Autodesk Inventor part; units mm, degrees
sketch "Sketch1" plane through (0, 0, 0) normal (0, 0, 1) x (1, 0, 0)
  line L0 (0, 1.6506) -> (0, -1.6506) construction
  line L1 (-3.3363, 0) -> (3.3363, 0) construction
  circle A0 centre (-22.86, -5.25) radius 2
  circle A1 centre (22.86, -5.25) radius 2
  circle A2 centre (0, 0) radius 2
  circle A3 centre (-35, -24) radius 2
  circle A4 centre (21, -24) radius 2
  circle A5 centre (35, -24) radius 2
  line L2 (-36.6788, -22.913) -> (-24.5388, -4.163)
  line L3 (-21.1812, -6.337) -> (-33.3212, -25.087)
  line L4 (33.3212, -25.087) -> (21.1812, -6.337)
  line L5 (24.5388, -4.163) -> (36.6788, -22.913)
  line L6 (23.3077, -3.3007) -> (0.4477, 1.9493)
  line L7 (-22.4123, -7.1993) -> (0.4477, -1.9493)
  line L8 (-23.3077, -3.3007) -> (-0.4477, 1.9493)
  line L9 (-0.4477, -1.9493) -> (22.4123, -7.1993)
  line L10 (19.0098, -23.8026) -> (20.8698, -5.0526)
  line L11 (22.9902, -24.1974) -> (24.8502, -5.4474)
  point P0 (19.0231, -24.3028)
  point P1 (1.0254, -1.7172)
  point P2 (-21.6219, -7.0177)
  point P3 (0, 3.0781)
  point P4 (22.9979, -23.9085)
  point P5 (21.6219, -7.0177)
  point P6 (24.2863, -11.1327)
  point P7 (20.6959, -6.8051)
  dimension "d0" = 45.72
  dimension "d1" = 22.86
  dimension "d4" = 4
  dimension "d5" = 4
  dimension "d6" = 4
  dimension "d7" = 18.75
  dimension "d8" = 18.75
  dimension "d9" = 14
  dimension "d10" = 18.75
  dimension "d11" = 56
  dimension "d12" = 70
  dimension "d13" = 35
  dimension "d14" = 4
  dimension "d15" = 4
  dimension "d16" = 4
  dimension "d34" = 5.25
  dimension "d35" = 5.25
extrude "Extrusion1" add sketch "Sketch1" along normal blind 2.4
sketch "Sketch2" plane through (0, 0, 2.4) normal (0, 0, 1) x (1, 0, 0)
  line L0 (-21.6219, -7.0177) -> (-33.3212, -25.087)
  arc A0 (-36.6788, -22.913) -> (-33.3212, -25.087) centre (-35, -24) ccw
  line L1 (-36.6788, -22.913) -> (-24.5388, -4.163)
  arc A1 (-23.3077, -3.3007) -> (-24.5388, -4.163) centre (-22.86, -5.25) ccw
  line L2 (-23.3077, -3.3007) -> (-0.4477, 1.9493)
  line L3 (24.5388, -4.163) -> (36.6788, -22.913)
  arc A2 (33.3212, -25.087) -> (36.6788, -22.913) centre (35, -24) ccw
  line L4 (33.3212, -25.087) -> (24.2863, -11.1327)
  line L5 (0, -2.0521) -> (-21.6219, -7.0177)
  arc A3 (19.0098, -23.8026) -> (22.9902, -24.1974) centre (21, -24) ccw
  line L6 (0.4477, 1.9493) -> (23.3077, -3.3007)
  arc A4 (24.5388, -4.163) -> (23.3077, -3.3007) centre (22.86, -5.25) ccw
  arc A5 (0.4477, 1.9493) -> (-0.4477, 1.9493) centre (0, 0) ccw
  line L7 (20.6959, -6.8051) -> (0, -2.0521)
  line L8 (24.2863, -11.1327) -> (22.9902, -24.1974)
  line L9 (19.0098, -23.8026) -> (20.6959, -6.8051)
hole "Hole1" at (-35, -24, 2.4) at (21, -24, 2.4) at (35, -24, 2.4) direction (0, 0, -1) diameter 2.8 depth 2.4
sketch "Sketch3" plane through (0, 0, 2.4) normal (0, 0, 1) x (1, 0, 0)
  circle A0 centre (35, -24) radius 1.4
  circle A1 centre (21, -24) radius 1.4
  circle A2 centre (-35, -24) radius 1.4
  line L0 (-21.6219, -7.0177) -> (-33.3212, -25.087)
  arc A3 (-36.6788, -22.913) -> (-33.3212, -25.087) centre (-35, -24) ccw
  line L1 (-36.6788, -22.913) -> (-24.5388, -4.163)
  arc A4 (-23.3077, -3.3007) -> (-24.5388, -4.163) centre (-22.86, -5.25) ccw
  line L2 (-23.3077, -3.3007) -> (-0.4477, 1.9493)
  line L3 (24.5388, -4.163) -> (36.6788, -22.913)
  arc A5 (33.3212, -25.087) -> (36.6788, -22.913) centre (35, -24) ccw
  line L4 (33.3212, -25.087) -> (24.2863, -11.1327)
  line L5 (0, -2.0521) -> (-21.6219, -7.0177)
  arc A6 (19.0098, -23.8026) -> (22.9902, -24.1974) centre (21, -24) ccw
  line L6 (0.4477, 1.9493) -> (23.3077, -3.3007)
  arc A7 (24.5388, -4.163) -> (23.3077, -3.3007) centre (22.86, -5.25) ccw
  arc A8 (0.4477, 1.9493) -> (-0.4477, 1.9493) centre (0, 0) ccw
  line L7 (20.6959, -6.8051) -> (0, -2.0521)
  line L8 (24.2863, -11.1327) -> (22.9902, -24.1974)
  line L9 (19.0098, -23.8026) -> (20.6959, -6.8051)
  circle A9 centre (-22.86, -5.25) radius 5
  circle A10 centre (0, 0) radius 4
  circle A11 centre (22.86, -5.25) radius 5
  dimension "d36" = 10
  dimension "d37" = 8
  dimension "d38" = 10
extrude "Extrusion3" add sketch "Sketch3" against normal up to surface (2.4 mm away) contours L5 A9 L0 | L0 A9 L1 A4 L2 L5 | A9 L2 A4 L1 | A10 L2 A8 L6 L7 L5 | L5 L7 A10 | A10 L6 A8 L2 | A11 L6 A7 L3 L9 L7 | L7 L9 A11 | A11 L3 A7 L6
sketch "Sketch4" plane through (0, 0, 0) normal (0, 0, -1) x (-1, 0, 0)
  arc A0 (-2.9285, -2.7246) -> (2.9285, -2.7246) centre (0, 0) ccw
  line L0 (-2.9285, -2.7246) -> (-17.946, -6.1735)
  arc A1 (-20.4174, -9.6128) -> (-17.946, -6.1735) centre (-22.86, -5.25) ccw
  line L1 (-20.4174, -9.6128) -> (-19.0098, -23.8026)
  arc A2 (-22.9902, -24.1974) -> (-19.0098, -23.8026) centre (-21, -24) ccw
  line L2 (-22.9902, -24.1974) -> (-24.2863, -11.1327)
  line L3 (-24.2863, -11.1327) -> (-33.3212, -25.087)
  arc A3 (-36.6788, -22.913) -> (-33.3212, -25.087) centre (-35, -24) ccw
  line L4 (-36.6788, -22.913) -> (-27.0294, -8.0097)
  arc A4 (-18.8414, -2.275) -> (-27.0294, -8.0097) centre (-22.86, -5.25) ccw
  line L5 (-18.8414, -2.275) -> (-3.8239, 1.1739)
  arc A5 (3.8239, 1.1739) -> (-3.8239, 1.1739) centre (0, 0) ccw
  line L6 (3.8239, 1.1739) -> (18.8414, -2.275)
  arc A6 (27.0294, -8.0097) -> (18.8414, -2.275) centre (22.86, -5.25) ccw
  line L7 (27.0294, -8.0097) -> (36.6788, -22.913)
  arc A7 (33.3212, -25.087) -> (36.6788, -22.913) centre (35, -24) ccw
  line L8 (33.3212, -25.087) -> (23.6718, -10.1837)
  arc A8 (17.946, -6.1735) -> (23.6718, -10.1837) centre (22.86, -5.25) ccw
  line L9 (17.946, -6.1735) -> (2.9285, -2.7246)
  circle A9 centre (-21, -24) radius 1.4
  circle A10 centre (-35, -24) radius 1.4
  circle A11 centre (35, -24) radius 1.4
hole "Hole3" at (-22.86, -5.25, 0) at (22.86, -5.25, 0) direction (0, 0, 1) diameter 3.3 depth 2.4 countersink diameter 6 countersink angle 90
sketch "Sketch5" plane through (0, 0, 2.4) normal (0, 0, 1) x (1, 0, 0)
  circle A0 centre (22.86, -5.25) radius 1.65
  circle A1 centre (-22.86, -5.25) radius 1.65
  arc A2 (-2.9285, -2.7246) -> (2.9285, -2.7246) centre (0, 0) ccw
  line L0 (-2.9285, -2.7246) -> (-17.946, -6.1735)
  arc A3 (-23.6718, -10.1837) -> (-17.946, -6.1735) centre (-22.86, -5.25) ccw
  line L1 (-23.6718, -10.1837) -> (-33.3212, -25.087)
  arc A4 (-36.6788, -22.913) -> (-33.3212, -25.087) centre (-35, -24) ccw
  line L2 (-36.6788, -22.913) -> (-27.0294, -8.0097)
  arc A5 (-18.8414, -2.275) -> (-27.0294, -8.0097) centre (-22.86, -5.25) ccw
  line L3 (-18.8414, -2.275) -> (-3.8239, 1.1739)
  arc A6 (3.8239, 1.1739) -> (-3.8239, 1.1739) centre (0, 0) ccw
  line L4 (3.8239, 1.1739) -> (18.8414, -2.275)
  arc A7 (27.0294, -8.0097) -> (18.8414, -2.275) centre (22.86, -5.25) ccw
  line L5 (27.0294, -8.0097) -> (36.6788, -22.913)
  arc A8 (33.3212, -25.087) -> (36.6788, -22.913) centre (35, -24) ccw
  line L6 (33.3212, -25.087) -> (24.2863, -11.1327)
  line L7 (24.2863, -11.1327) -> (22.9902, -24.1974)
  arc A9 (19.0098, -23.8026) -> (22.9902, -24.1974) centre (21, -24) ccw
  line L8 (19.0098, -23.8026) -> (20.4174, -9.6128)
  arc A10 (17.946, -6.1735) -> (20.4174, -9.6128) centre (22.86, -5.25) ccw
  line L9 (17.946, -6.1735) -> (2.9285, -2.7246)
  circle A11 centre (21, -24) radius 1.4
  circle A12 centre (35, -24) radius 1.4
  circle A13 centre (-35, -24) radius 1.4
hole "Hole4" at (0, 0, 2.4) direction (0, 0, -1) diameter 3.3 depth 2.4
properties part number "PD_Sensor" material "S235"
Design review of the part built by this model. Coordinates are the model's own, in mm. A direction names the side the tool comes from. Give positions to 0.01 mm unless a question says otherwise; leave off trailing zeros. Write each loop counter-clockwise with the first axis right and the second up, starting at its lowest first coordinate (ties: lowest second). Pieces come first, ordered by that corner, then holes.
(1) Mouldability with a two-part tool opening along X and no side actions: class faces 4 (the face through (31.79, -15.36, 1.18)), 5 (the face through (-31.922, -15.566, 1.183)), 6 (the face through (10.332, -4.425, 1.183)), 7 (the face through (-10.542, -4.473, 1.183)) as +X half, -X half, draft (parallel to the pull), parting line (faces both ways), or undercut.
Checked values:
face 4: +X half
face 5: -X half
face 6: undercut
face 7: undercut
(2) Add section B-B (x = -22.86). Give the boundary of the cut face in (y, z).
Checked values:
outline: (-10.25, 0) - (-8.25, 0) - (-6.9, 1.35) - (-6.9, 2.4) - (-10.25, 2.4) - close; (-3.6, 1.35) - (-2.25, 0) - (-0.25, 0) - (-0.25, 2.4) - (-3.6, 2.4) - close
(3) Tool access review of faces 1 (the face through (18.78, -8.14, 1.22)), 2 (the face through (-28.43, -17.53, 1.18)), 3 (the face through (11.438, -0.575, 1.183)): name each direction out of +Z, -Z, +X, -X, +Y, -Y from which nothing blocks a thin tool from reaching the whole face with its end or side.
Checked values:
face 1: +Z, -Z
face 2: +Z, -Z, -Y
face 3: +Z, -Z, +Y
(4) Wall thickness on line 1 along X through (y, z) = (-24, 1.9); line 2 along Y through (x, z) = (-22.86, 2.1); line 3 along X through (y, z) = (-22, 0.7): over which ranges is each line inside the solid? List them lowest first.
Checked values:
line 1: x = -37 to -36.4, -33.6 to -32.62, 19 to 19.6, 22.4 to 23.01, 32.62 to 33.6, 36.4 to 37
line 2: y = -10.25 to -6.9, -3.6 to -0.25
line 3: x = -36.09 to -31.32, 19.19 to 23.21, 31.32 to 36.09
(5) Add section D-D (y = -5.25). Give the boundary of the cut face in (x, z), and give its area (3 significant figures).
Checked values:
outline: (-27.86, 0) - (-25.86, 0) - (-24.51, 1.35) - (-24.51, 2.4) - (-27.86, 2.4) - close; (-21.21, 1.35) - (-19.86, 0) - (-13.92, 0) - (-13.92, 2.4) - (-21.21, 2.4) - close; (13.92, 0) - (19.86, 0) - (21.21, 1.35) - (21.21, 2.4) - (13.92, 2.4) - close; (24.51, 1.35) - (25.86, 0) - (27.86, 0) - (27.86, 2.4) - (24.51, 2.4) - close
area: 47.4 mm2
(6) Add section C-C (z = 0.5). Give the boundary of the cut face in (x, y).
Checked values:
outline: (-36.68, -22.91) arc R2 ccw to (-33.32, -25.09) - (-23.67, -10.18) arc R5 ccw to (-17.95, -6.17) - (-2.93, -2.72) arc R4 ccw to (2.93, -2.72) - (17.95, -6.17) arc R5 ccw to (20.42, -9.61) - (19.01, -23.8) arc R2 ccw to (22.99, -24.2) - (24.29, -11.13) - (33.32, -25.09) arc R2 ccw to (36.68, -22.91) - (27.03, -8.01) arc R5 ccw to (18.84, -2.27) - (3.82, 1.17) arc R4 ccw to (-3.82, 1.17) - (-18.84, -2.27) arc R5 ccw to (-27.03, -8.01) - close; hole circle Ø2.8 at (-35, -24); hole circle Ø5 at (-22.86, -5.25); hole circle Ø3.3 at (0, 0); hole circle Ø2.8 at (21, -24); hole circle Ø5 at (22.86, -5.25); hole circle Ø2.8 at (35, -24)
(7) Clearance check with flat-ended pins moving along their axes: pin 1 Ø4 at (x, y) = (22.86, -5.25) entering from -Z; pin 2 Ø2.5 at (x, y) = (-22.86, -5.25) entering from +Z. State where each tip first meets the part, or that it passes through.
Checked values:
pin 1: stops at z = 1
pin 2: passes through
(8) Add section A-A (y = -21.75). Give the boundary of the cut face in (x, z), and give its area (3 significant figures).
Checked values:
outline: (-35.93, 0) - (-31.16, 0) - (-31.16, 2.4) - (-35.93, 2.4) - close; (19.21, 0) - (23.23, 0) - (23.23, 2.4) - (19.21, 2.4) - close; (31.16, 0) - (35.93, 0) - (35.93, 2.4) - (31.16, 2.4) - close
area: 32.5 mm2
